Could you check a few things on this model? Use its own coordinates, in mm. A direction names the side the tool comes from. Give positions to 0.01 mm unless a question says otherwise; leave off trailing zeros. Loops run counter-clockwise (first coordinate to the right, second up) from the corner with the lowest first, then second, coordinate; pieces in that order, holes last.
1. Imagine slicing it at A-A (x = 0). List the corners of the cut face in (y, z) for me.
2. Imagine slicing it at C-C (y = -7.3). List the corners of the cut face in (x, z) for me, plus the area to 3 significant figures.
3. For P1, Ø3.5, axis at x = 6.32, y = 3.65, coming from the +Z side; P2, Ø1.5, axis at y = -32.5, z = 2, coming from the +X side; P3, Ø1.5, axis at x = 12.5, z = 4.5, coming from the +Y side; P4, Ø10, axis at x = 9.5, y = -1, coming from the -Z side, each with a flat end and sliding along its axis, tell me the tip position at first contact or that it passes through.
4. Thinking about a two-plate mould opening in Z: for faces 4 (the flat face through (1, -10, 6)), 5 (the cylindrical face through (-13.55, -32.52, 1.57)), 6 (the flat face through (-14.534, -14.988, 4.291)), which applies, +Z half, -Z half, draft (parallel to the pull), parting line (faces both ways), or undercut?
5. Imagine slicing it at D-D (y = -25.5). List the corners of the cut face in (x, z) for me, plus the area to 3 significant figures.
6. Imagine slicing it at B-B (y = 0). List the corners of the cut face in (x, z) for me, plus the area to 3 significant figures.
7. For faces 1 (the flat face through (4, -31, 1)), 2 (the cylindrical face through (24.265, -32.521, 2.194)), 3 (the cylindrical face through (-7.85, -8.354, 4.479)), which set-ups out of +Z, -Z, +X, -X, +Y, -Y let a thin tool reach every point of the face, with its end or its side?
8. I need wall thicknesses on line 1 along Y through (x, z) = (0, 4.9); line 2 along X through (y, z) = (3.65, 4.15); line 3 along X through (y, z) = (-3.65, 5). Which ranges of each line are inside material? Lowest first, please.
```python
from build123d import *

# Parameters (mm, degrees)
SKETCH_1_R          = 4
SKETCH_1_R_2        = 1.5
EXTRUDE_1_DEPTH     = 6
SKETCH_4_R          = 1.5
CUT_EXTRUDE_2_DEPTH = 3
CUT_EXTRUDE_3_DEPTH = 3


with BuildPart() as part:
    # 草图1 → 凸台-拉伸1 (new body)
    with BuildSketch(Plane.XY):
        with BuildLine():
            Line((-10.191413347, 2.526874351), (-19, -33))
            Line((-19, -33), (-19, -34))
            Line((-19, -34), (33, -34))
            Line((33, -34), (33, -33))
            Line((33, -33), (8.904718959, 5.563809869))
            ThreePointArc((8.904718959, 5.563809869), (-1.649133089, 10.369684665), (-10.191413347, 2.526874351))
        make_face()
        Circle(SKETCH_1_R, mode=Mode.SUBTRACT)
        with Locations((0, 7.3)):
            Circle(SKETCH_1_R_2, mode=Mode.SUBTRACT)
        with Locations((6.321985448, 3.65)):
            Circle(SKETCH_1_R_2, mode=Mode.SUBTRACT)
        with Locations((6.321985448, -3.65)):
            Circle(SKETCH_1_R_2, mode=Mode.SUBTRACT)
        with Locations((0, -7.3)):
            Circle(SKETCH_1_R_2, mode=Mode.SUBTRACT)
        with Locations((-6.321985448, -3.65)):
            Circle(SKETCH_1_R_2, mode=Mode.SUBTRACT)
        with Locations((-6.321985448, 3.65)):
            Circle(SKETCH_1_R_2, mode=Mode.SUBTRACT)
        with BuildLine():
            Line((-9.115462127, -9.754914157), (-13.519839571, -27.5186906))
            ThreePointArc((-13.519839571, -27.5186906), (-13.153835237, -29.232351654), (-11.578617982, -30))
            Line((-11.578617982, -30), (22.801020138, -30))
            ThreePointArc((22.801020138, -30), (24.55024091, -28.969652872), (24.497157083, -26.940226692))
            Line((24.497157083, -26.940226692), (11.69193225, -6.445829679))
            ThreePointArc((11.69193225, -6.445829679), (10.081363796, -5.507434318), (8.396468057, -6.30470651))
            ThreePointArc((8.396468057, -6.30470651), (1.649133089, -10.369684665), (-6.026362051, -8.598427788))
            ThreePointArc((-6.026362051, -8.598427788), (-7.875463398, -8.363181513), (-9.115462127, -9.754914157))
        make_face(mode=Mode.SUBTRACT)
    extrude(amount=EXTRUDE_1_DEPTH)

    # 草图4 → 切除-拉伸2 (cut)
    with BuildSketch(Plane(origin=(0, -34, 0), x_dir=(-1, 0, 0), z_dir=(0, -1, 0))):
        with Locations(Location((14, -3, 0), (0, 0, 90))):
            Circle(SKETCH_4_R)
        with Locations(Location((-23, -3, 0), (0, 0, 90))):
            Circle(SKETCH_4_R)
    extrude(amount=-CUT_EXTRUDE_2_DEPTH, mode=Mode.SUBTRACT)

    # 草图5 → 切除-拉伸3 (cut)
    with BuildSketch(Plane(origin=(0, 0, 0), x_dir=(-1, 0, 0), z_dir=(0, 0, -1))):
        Polygon((22.848175367, -31), (-28, -31), (-28, -36.198371548), (-37.735885528, -36.198371548), (-37.735885528, 13.676691154), (23.360590395, 13.676691154), (23.360590395, -30.988818766), align=None)
    extrude(amount=-CUT_EXTRUDE_3_DEPTH, mode=Mode.SUBTRACT)


solid = part.part
```
Derived:
1. outline: (-34, 0) - (-31, 0) - (-31, 3) - (-30, 3) - (-30, 6) - (-34, 6) - close; (-10.5, 3) - (-8.8, 3) - (-8.8, 6) - (-10.5, 6) - close; (-5.8, 3) - (-4, 3) - (-4, 6) - (-5.8, 6) - close; (4, 3) - (5.8, 3) - (5.8, 6) - (4, 6) - close; (8.8, 3) - (10.5, 3) - (10.5, 6) - (8.8, 6) - close
2. outline: (-12.63, 3) - (-1.5, 3) - (-1.5, 6) - (-12.63, 6) - close; (1.5, 3) - (7.55, 3) - (7.55, 6) - (1.5, 6) - close; (12.23, 3) - (16.94, 3) - (16.94, 6) - (12.23, 6) - close
2. area: 65.7 mm2
3. P1: stops at z = 6
3. P2: stops at x = 28
3. P3: stops at y = 1.01
3. P4: stops at z = 3
4. face 4: +Z half
4. face 5: undercut
4. face 6: draft
5. outline: (-17.14, 3) - (-13.02, 3) - (-13.02, 6) - (-17.14, 6) - close; (23.6, 3) - (28.31, 3) - (28.31, 6) - (23.6, 6) - close
5. area: 26.5 mm2
6. outline: (-10.82, 3) - (-4, 3) - (-4, 6) - (-10.82, 6) - close; (4, 3) - (12.38, 3) - (12.38, 6) - (4, 6) - close
6. area: 45.6 mm2
7. face 1: -Z, +X, -X, +Y
7. face 2: -Y
7. face 3: +Z, -Z
8. line 1: y = -34 to -30, -10.5 to -8.8, -5.8 to -4, 4 to 5.8, 8.8 to 10.5
8. line 2: x = -9.85 to -7.82, -4.82 to -1.64, 1.64 to 4.82, 7.82 to 10.1
8. line 3: x = -11.72 to -7.82, -4.82 to -1.64, 1.64 to 4.82, 7.82 to 14.66
